Input: dimensioned drawing with shaded views. Units: mm. Origin: part minimum x, y, z. A direction names the side the tool comes from. Give positions to 0.01 mm unless a question says otherwise; leave off trailing zeros. Loops run counter-clockwise (first coordinate to the right, second up) from the corner with the lowest first, then second, coordinate; pieces in that order, holes last. Notation, with made-up numbers: (31.25, 61.5) -> (49.25, 61.5) arc R21 cw to (49.25, 75.5) -> close; hole circle Ø4 at (-29.5, 89.5). An arc over 180 degrees is marked (long way). One line per question, with ' | ' between items. Start each with the question number.
Item 1: Set-up query: the marked faces 1 and 2. Return all of +Z, -Z, +X, -X, +Y, -Y with unobstructed straight access to the full face (end or side cutting, diameter ignored); none if empty.
Item 2: Section D-D on y = 39. Return loops of the section in (x, z).
Item 3: Material intervals for line 1 along X through (y, z) = (29.5, 6.5) (1 decimal); line 2 along X through (y, z) = (6, 9.25); line 3 along Y through (x, z) = (112, 8), sorted ascending. Write a range as [from, to].
Item 4: Section C-C on y = 33.5. Return loops of the section in (x, z), then the cut area to 3 significant figures.
Item 5: Mould query, pull axis X, two halves, no side actions, for the marked faces 3, 4 and 5. Classes: released by +X, released by -X, zero draft, split by the parting line, or undercut.
Item 6: Pin query (flat end, axial travel): P1, Ø5, axis at y = 5, z = 6.5, coming from the -X side; P2, Ø1.5, axis at y = 24, z = 6.5, coming from the +X side; P3, Ø4, axis at y = 15.5, z = 8, coming from the -X side. Return the tip coordinate at first contact, or that it passes through.
Item 7: Section B-B on z = 8. Return loops of the section in (x, y) (3 decimals).
Item 8: Section A-A on x = 18. Return loops of the section in (y, z), then the cut area to 3 significant figures.
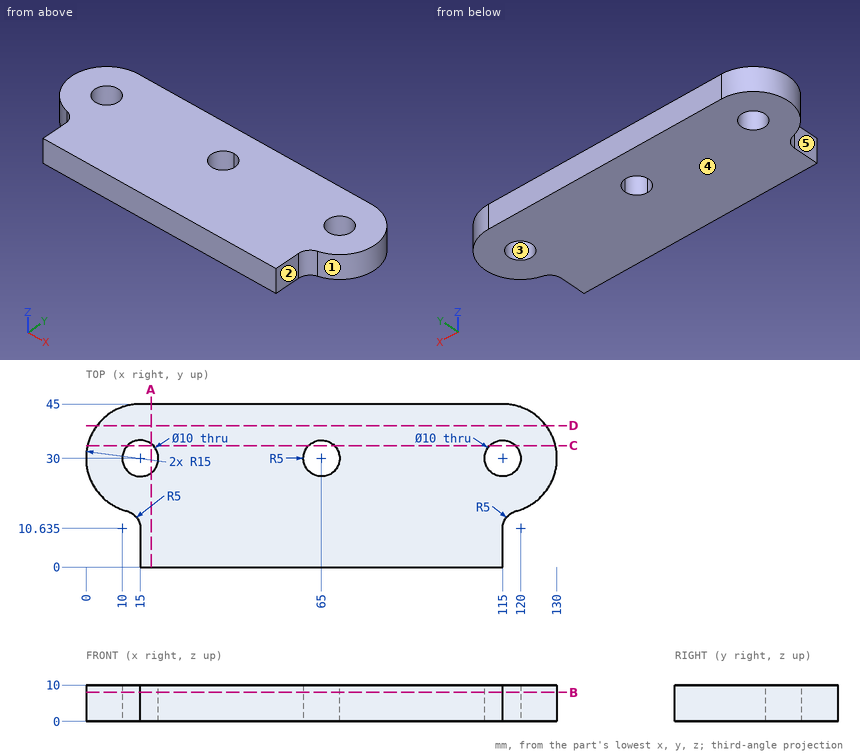
Result sheet:
1) face 1: +Z, -Z, +X | face 2: +Z, -Z, +X, -Y
2) outline: (3, 0) -> (127, 0) -> (127, 10) -> (3, 10) -> close
3) line 1: x = [0, 10], [20, 60], [70, 110], [120, 130] | line 2: x = [15, 115] | line 3: y = [0, 26], [34, 45]
4) outline: (0.41, 0) -> (11.43, 0) -> (11.43, 10) -> (0.41, 10) -> close; (18.57, 0) -> (61.43, 0) -> (61.43, 10) -> (18.57, 10) -> close; (68.57, 0) -> (111.43, 0) -> (111.43, 10) -> (68.57, 10) -> close; (118.57, 0) -> (129.59, 0) -> (129.59, 10) -> (118.57, 10) -> close | area: 1,080 mm²
5) face 3: undercut | face 4: zero draft | face 5: released by -X
6) P1: stops at x = 15 | P2: stops at x = 129.05 | P3: stops at x = 6.71
7) outline: (11.25, 15.476) arc R5 cw to (15, 10.635) -> (15, 0) -> (115, 0) -> (115, 10.635) arc R5 cw to (118.75, 15.476) arc R15 ccw to (115, 45) -> (15, 45) arc R15 ccw to start; hole circle Ø10 at (15, 30); hole circle Ø10 at (65, 30); hole circle Ø10 at (115, 30)
8) outline: (0, 0) -> (26, 0) -> (26, 10) -> (0, 10) -> close; (34, 0) -> (45, 0) -> (45, 10) -> (34, 10) -> close | area: 370 mm²
